```python
from build123d import *

# Parameters (mm, degrees)
SKETCH1_W           = 48
SKETCH1_H           = 23
BOSS_EXTRUDE1_DEPTH = 100
SKETCH2_W           = 48
SKETCH2_H           = 10
CUT_EXTRUDE1_DEPTH  = 5
SKETCH3_R           = 39
BOSS_EXTRUDE2_DEPTH = 45
BOSS_EXTRUDE2_DRAFT = -2.5
SKETCH6_R           = 27.964742431
CUT_EXTRUDE3_DEPTH  = 55
CUT_EXTRUDE3_DRAFT  = -2.5
SKETCH9_R           = 39
BOSS_EXTRUDE4_DEPTH = 10
CUT_EXTRUDE5_REACH  = 158.762
SKETCH11_W          = 38
SKETCH11_H          = 13
SKETCH12_R          = 1.5
BOSS_EXTRUDE5_DEPTH = 2
REVOLVE1_START      = 46
REVOLVE1_DEPTH      = 9
REVOLVE1_START_2    = 55
REVOLVE1_2_DEPTH    = 9
CIRPATTERN1_COUNT   = 3
SKETCH15_R          = 50.01
CUT_EXTRUDE6_DEPTH  = 75
CUT_EXTRUDE8_REACH  = 169.525
SKETCH17_R          = 38.964742431
SKETCH18_W          = 27
SKETCH18_H          = 25.5
BOSS_EXTRUDE6_DEPTH = 45
SKETCH19_W          = 27
SKETCH19_H          = 5
BOSS_EXTRUDE7_DEPTH = 6
SKETCH20_W          = 25
SKETCH20_H          = 5
CUT_EXTRUDE9_DEPTH  = 4
SKETCH21_W          = 21
SKETCH21_H          = 2.5
CUT_EXTRUDE10_DEPTH = 119.502093026
SKETCH22_W          = 2
SKETCH22_H          = 10
BOSS_EXTRUDE8_DEPTH = 3
SKETCH23_W          = 1
SKETCH23_H          = 2
CUT_EXTRUDE11_DEPTH = 14


# Read off the part's stored shape, not the designer's step: Revolve1
with BuildPart() as part:
    # Sketch1 → Boss-Extrude1 (new body)
    with BuildSketch(Plane.XY):
        with Locations((0, 11.5)):
            Rectangle(SKETCH1_W, SKETCH1_H)
    extrude(amount=BOSS_EXTRUDE1_DEPTH)

    # Sketch2 → Cut-Extrude1 (cut)
    with BuildSketch(Plane.XY):
        with Locations((0, 5)):
            Rectangle(SKETCH2_W, SKETCH2_H)
    extrude(amount=CUT_EXTRUDE1_DEPTH, mode=Mode.SUBTRACT)


with BuildPart() as boss_extrude2_tool:
    # Sketch3 → Boss-Extrude2 (with draft: the straight prism first)
    with BuildSketch(Plane(origin=(0, 10, 0), x_dir=(-1, 0, 0), z_dir=(0, 1, 0))):
        with Locations((0, 100)):
            Circle(SKETCH3_R)
    extrude(amount=BOSS_EXTRUDE2_DEPTH)
    # Boss-Extrude2: the draft: its side faces are tilted about the plane it starts from
    boss_extrude2_sides = [boss_extrude2_tool.faces().sort_by_distance(p)[0] for p in [
        (39, 32.5, 100),
    ]]
    draft(boss_extrude2_sides, Plane(origin=(0, 10, 0), x_dir=(-1, 0, 0), z_dir=(0, 1, 0)), BOSS_EXTRUDE2_DRAFT)


with BuildPart() as part_1:
    add(part.part)

    # Boss-Extrude2: add boss_extrude2_tool
    add(boss_extrude2_tool.part)


with BuildPart() as cut_extrude3_tool:
    # Sketch6 → Cut-Extrude3 (with draft: the straight prism first)
    with BuildSketch(Plane(origin=(0, 55, 0), x_dir=(1, 0, 0), z_dir=(0, 1, 0))):
        with Locations((0, -100)):
            Circle(SKETCH6_R)
    extrude(amount=-CUT_EXTRUDE3_DEPTH)
    # Cut-Extrude3: the draft: its side faces are tilted about the plane it starts from
    cut_extrude3_sides = [cut_extrude3_tool.faces().sort_by_distance(p)[0] for p in [
        (-27.964742431, 27.5, 100),
    ]]
    draft(cut_extrude3_sides, Plane(origin=(0, 55, 0), x_dir=(1, 0, 0), z_dir=(0, 1, 0)), CUT_EXTRUDE3_DRAFT)


with BuildPart() as part_2:
    add(part_1.part)

    # Cut-Extrude3: cut by cut_extrude3_tool
    add(cut_extrude3_tool.part, mode=Mode.SUBTRACT)

    # Sketch9 → Boss-Extrude4 (add)
    with BuildSketch(Plane.XZ.offset(-10)):
        with Locations((0, 100)):
            Circle(SKETCH9_R)
    extrude(amount=BOSS_EXTRUDE4_DEPTH)

    # Cut-Extrude5: up to this cone (the profile starts outside it)
    cut_extrude5_end = Plane(origin=(0, 11.5, 100), z_dir=(0, 1, 0)) * Cone(17.973918392, 34.157064436, 370.654982829, mode=Mode.PRIVATE)
    # Sketch11 → Cut-Extrude5 (cut, up to the surface)
    with BuildSketch(Plane(origin=(0, 0, 0), x_dir=(-1, 0, 0), z_dir=(0, 0, -1)), mode=Mode.PRIVATE) as cut_extrude5_sk1:
        with Locations((0, 11.5)):
            Rectangle(SKETCH11_W, SKETCH11_H)
    cut_extrude5_tool1 = extrude(cut_extrude5_sk1.sketch, amount=-CUT_EXTRUDE5_REACH, mode=Mode.PRIVATE) - cut_extrude5_end
    add(cut_extrude5_tool1.solids().sort_by_distance((0, 11.5, 0))[0], mode=Mode.SUBTRACT)

    # Sketch12 → Boss-Extrude5 (add)
    with BuildSketch(Plane(origin=(0, 55, 0), x_dir=(1, 0, 0), z_dir=(0, 1, 0))):
        with Locations(Location((32, -100, 0), (0, 0, 90))):
            Circle(SKETCH12_R)
        with Locations(Location((-32, -100, 0), (0, 0, 270))):
            Circle(SKETCH12_R)
    extrude(amount=BOSS_EXTRUDE5_DEPTH)

    # Revolve1 outline → Revolve1 (add)
    with BuildSketch(Plane(origin=(0, 0, 0), x_dir=(1, 0, 0), z_dir=(0, 1, 0)).offset(REVOLVE1_START)):
        with BuildLine():
            Line((-3.536064836, -140.41740602), (-4.468016703, -151.069664609))
            ThreePointArc((-4.468016703, -151.069664609), (0, -151.264742431), (4.468016703, -151.069664609))
            Line((4.468016703, -151.069664609), (3.536064836, -140.41740602))
            Line((3.536064836, -140.41740602), (3.499546541, -140))
            Line((3.499546541, -140), (-3.499546541, -140))
            Line((-3.499546541, -140), (-3.536064836, -140.41740602))
        make_face()
    revolve1 = extrude(amount=REVOLVE1_DEPTH)

    # Revolve1 2 outline → Revolve1 2 (add)
    with BuildSketch(Plane(origin=(0, 0, 0), x_dir=(1, 0, 0), z_dir=(0, 1, 0)).offset(REVOLVE1_START_2)):
        with BuildLine():
            ThreePointArc((4.293705218, -149.077275213), (0, -149.264742431), (-4.293705218, -149.077275213))
            Line((-4.293705218, -149.077275213), (-4.468016703, -151.069664609))
            ThreePointArc((-4.468016703, -151.069664609), (0, -151.264742431), (4.468016703, -151.069664609))
            Line((4.468016703, -151.069664609), (4.293705218, -149.077275213))
        make_face()
    revolve1_2 = extrude(amount=REVOLVE1_2_DEPTH)

    # CirPattern1: Revolve1, Revolve1 2 ×3 about axis
    cirpattern1_axis = Axis((0, 0, 100), (0, 1, 0))
    add([revolve1.rotate(cirpattern1_axis, i * 360 / CIRPATTERN1_COUNT) for i in range(1, CIRPATTERN1_COUNT)])
    add([revolve1_2.rotate(cirpattern1_axis, i * 360 / CIRPATTERN1_COUNT) for i in range(1, CIRPATTERN1_COUNT)])

    # Sketch15 → Cut-Extrude6 (cut)
    with BuildSketch(Plane(origin=(0, 130, 0), x_dir=(1, 0, 0), z_dir=(0, 1, 0))):
        with Locations((0, -100)):
            Circle(SKETCH15_R)
    extrude(amount=-CUT_EXTRUDE6_DEPTH, mode=Mode.SUBTRACT)

    # Cut-Extrude8: up to this face of the body (flat: up to its plane)
    cut_extrude8_end = Plane(part_2.part.faces().sort_by_distance((0, 10, 100))[0])
    # Sketch17 → Cut-Extrude8 (cut, up to the picked face)
    with BuildSketch(Plane(origin=(0, 55, 0), x_dir=(1, 0, 0), z_dir=(0, 1, 0)), mode=Mode.PRIVATE) as cut_extrude8_sk1:
        with Locations(Location((0, -100, 0), (0, 0, 270))):
            Circle(SKETCH17_R)
    cut_extrude8_tool1 = split(extrude(cut_extrude8_sk1.sketch, amount=-CUT_EXTRUDE8_REACH, mode=Mode.PRIVATE), bisect_by=cut_extrude8_end, keep=Keep.BOTH, mode=Mode.PRIVATE)
    add(cut_extrude8_tool1.solids().sort_by(Axis((0, 55, 100), (0, -1, 0)))[0], mode=Mode.SUBTRACT)

    # Sketch18 → Boss-Extrude6 (add)
    with BuildSketch(Plane(origin=(0, 10, 0), x_dir=(1, 0, 0), z_dir=(0, 1, 0))):
        with Locations((0, -100)):
            Rectangle(SKETCH18_W, SKETCH18_H)
    extrude(amount=BOSS_EXTRUDE6_DEPTH)

    # Sketch19 → Boss-Extrude7 (add)
    with BuildSketch(Plane(origin=(0, 55, 0), x_dir=(1, 0, 0), z_dir=(0, 1, 0))):
        with Locations((0, -89.75)):
            Rectangle(SKETCH19_W, SKETCH19_H)
    extrude(amount=BOSS_EXTRUDE7_DEPTH)

    # Sketch20 → Cut-Extrude9 (cut)
    with BuildSketch(Plane.XY.offset(92.25)):
        with Locations((0, 57.5)):
            Rectangle(SKETCH20_W, SKETCH20_H)
    extrude(amount=-CUT_EXTRUDE9_DEPTH, mode=Mode.SUBTRACT)

    # Sketch21 → Cut-Extrude10 (cut, through all)
    with BuildSketch(Plane.XY.offset(88.25)):
        with Locations((0, 57.75)):
            Rectangle(SKETCH21_W, SKETCH21_H)
    extrude(amount=-CUT_EXTRUDE10_DEPTH, mode=Mode.SUBTRACT)

    # Sketch22 → Boss-Extrude8 (add)
    with BuildSketch(Plane(origin=(0, 55, 0), x_dir=(1, 0, 0), z_dir=(0, 1, 0))):
        with Locations((-12.5, -97.25)):
            Rectangle(SKETCH22_W, SKETCH22_H)
        with Locations((12.5, -97.25)):
            Rectangle(SKETCH22_W, SKETCH22_H)
    extrude(amount=BOSS_EXTRUDE8_DEPTH)

    # Sketch23 → Cut-Extrude11 (cut)
    with BuildSketch(Plane.XY.offset(102.25)):
        with Locations((12, 56)):
            Rectangle(SKETCH23_W, SKETCH23_H)
        with Locations((-12, 56)):
            Rectangle(SKETCH23_W, SKETCH23_H)
    extrude(amount=-CUT_EXTRUDE11_DEPTH, mode=Mode.SUBTRACT)


solid = part_2.part
```
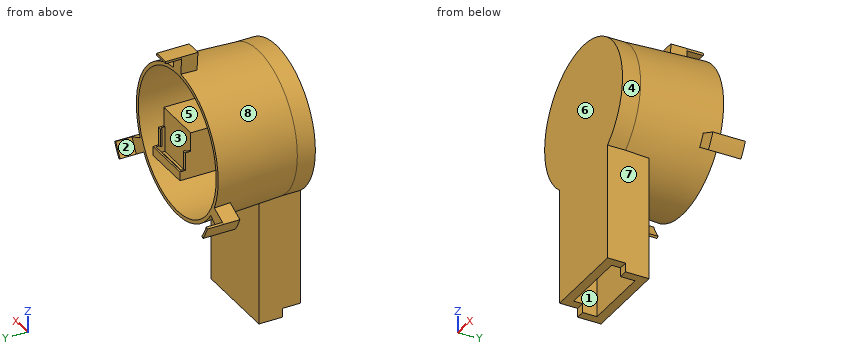
The listing builds one solid part. Answer for the finished solid, in the listing's coordinates (mm). Face numbers are marked on the shaded views. A direction names the side the tool comes from. Give positions to 0.01 mm unless a question says otherwise; leave off trailing zeros. Order: outer loops, then holes, each group sorted by start corner. A loop starts at its lowest first (then second) coordinate and runs counter-clockwise, first axis right, second up. Notation, with made-up numbers: (81, -32.75) -> (96, -32.75) arc R18 cw to (96, -26.75) -> close; hole circle Ø1 at (70.5, 72). An arc over 180 degrees is marked (long way). Answer as CSV lines item,"result". Start each with the question number.
Q1. A cutting plane is placed at D-D (z = 100). Determine the outline of the cut face in (x, y), then the cut area to 3 significant figures.
Q2. A cutting plane is placed at C-C (y = 41). Determine the outline of the cut face in (x, z).
Q3. Determine the mould class of the marked faces 6, 7 and 8 for opening direction Y: pulls with the +Y half, pulls with the -Y half, needs draft (parallel to the pull), parting line crosses it, or undercut.
Q4. Given pin 1 (10 mm diameter, centred on x = -2, z = 147, fed in from -Y); pin 2 (14.5 mm diameter, centred on y = 10, z = 43, fed in from -X); pin 3 (2.5 mm diameter, centred on x = -22.5, z = 1.5, fed in from -Y); pin 4 (8 mm diameter, centred on x = 1.5, y = 43.5, fed in from +Z), each flat-ended and moving along its own axis, determine where each tip first touches the part or whether it passes through.
Q5. Which of the six approach directions +Z, -Z, +X, -X, +Y, -Y give full straight-line access (tool end or side, diameter ignored) to the marked faces 1, 2, 3, 4 and 5?
Q6. A cutting plane is placed at B-B (z = 26.5). Determine the outline of the cut face in (x, y).
Q7. Find the intervals of material crossed by L1, parallel to X at y = 39, z = 100; L2, parallel to Y at x = 9, z = 31; L3, parallel to X at y = 21.5, z = 100, in increasing order.
Q8. A cutting plane is placed at A-A (x = 0). Count the separate pieces of the cut face and the enclosed holes in it, then the cut area to 3 significant figures.
Results found:
1,outline,"(-40.96, 55) -> (-39, 10) -> (-39, 0) -> (39, 0) -> (39, 10) -> (40.96, 55) -> (38.96, 55) -> (38.96, 10) -> (13.5, 10) -> (13.5, 58) -> (11.5, 58) -> (11.5, 57) -> (12.5, 57) -> (12.5, 55) -> (-12.5, 55) -> (-12.5, 57) -> (-11.5, 57) -> (-11.5, 58) -> (-13.5, 58) -> (-13.5, 10) -> (-38.96, 10) -> (-38.96, 55) -> close"
1,area,"2,090 mm2"
2,outline,"circle Ø80.71 at (0, 100); (-13.5, 87.25) -> (13.5, 87.25) -> (13.5, 112.75) -> (-13.5, 112.75) -> close; hole circle Ø77.93 at (0, 100)"
3,face 6,"pulls with the -Y half"
3,face 7,"needs draft"
3,face 8,"undercut"
4,pin 1,"y = 46"
4,pin 2,"x = -24"
4,pin 3,"y = 10"
4,pin 4,"z = 151.26"
5,face 1,"-Z"
5,face 2,"+Z, +Y"
5,face 3,"none"
5,face 4,"-Y"
5,face 5,"+Y"
6,outline,"(-24, 0) -> (24, 0) -> (24, 23) -> (-24, 23) -> close; hole (-19, 5) -> (19, 5) -> (19, 18) -> (-19, 18) -> close"
7,L1,"-40.27 to -38.96, -13.5 to 13.5, 38.96 to 40.27"
7,L2,"0 to 5, 18 to 23"
7,L3,"-39.5 to -38.96, -13.5 to 13.5, 38.96 to 39.5"
8,separate pieces,"3"
8,enclosed holes,"0"
8,area,"2,650 mm2"
